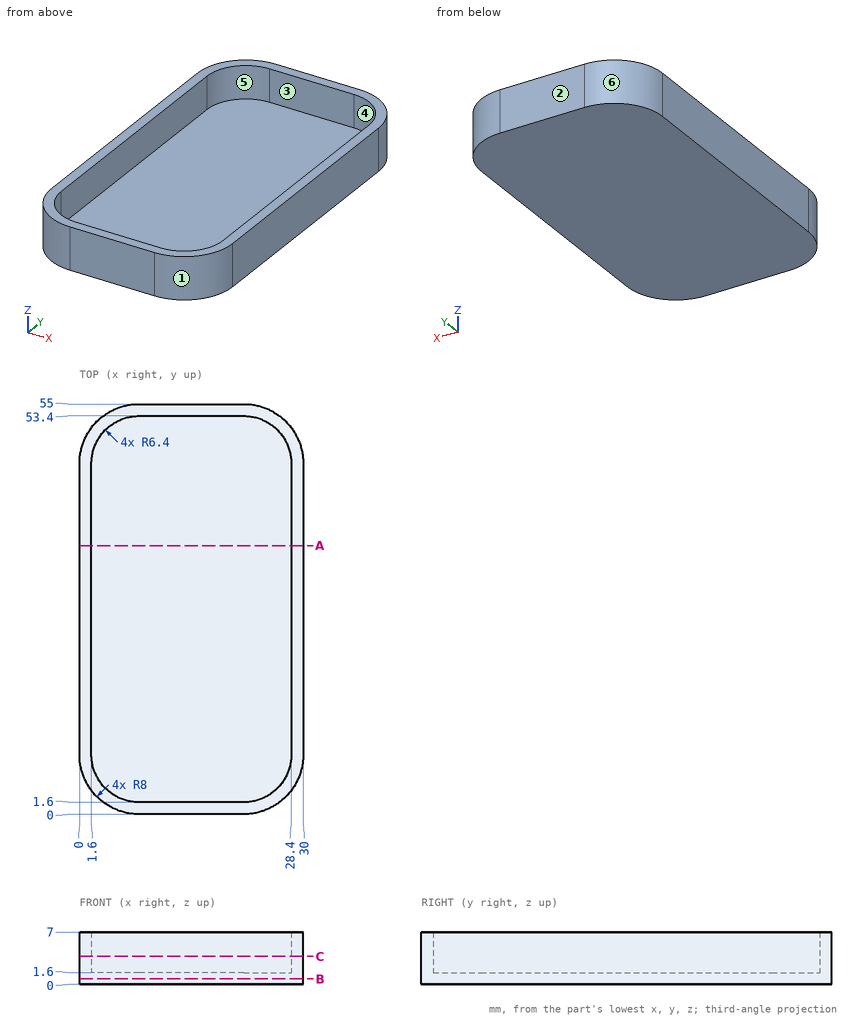
For this review, use the dimensioned drawing (mm, ordinates from the lowest corner) and the shaded views. A direction names the side the tool comes from. Round coordinates to 2 decimals unless told otherwise and drop trailing zeros. Write each loop counter-clockwise with the first axis right and the second up, starting at its lowest first coordinate (ties: lowest second). Pieces come first, ordered by that corner, then holes. Notation, with made-up numbers: (13.25, 46.25) -> (59.25, 46.25) arc R10 ccw to (59.25, 53.25) -> close; hole circle Ø11 at (-24, 75). An arc over 180 degrees is marked (long way). Use CSV: the item, a comma, the result in double quotes.
(1) Draft analysis for pull direction Y (two halves, no side actions). For the marked faces 1, 2, 3 and 4, state which applies: +Y half, -Y half, draft (parallel to the pull), parting line (faces both ways), or undercut.
Computed values:
face 1,"-Y half"
face 2,"+Y half"
face 3,"undercut"
face 4,"undercut"
(2) For the marked faces 5 and 6, list the 3-axis set-ups (+Z, -Z, +X, -X, +Y, -Y) from which the entire face can be reached by the end or side of a thin tool; tool diameter is ignored.
Computed values:
face 5,"+Z"
face 6,"+Z, -Z, -X, +Y"
(3) Consider section A-A, the plane y = 36. Give the boundary of the cut face in (x, z).
Computed values:
outline,"(0, 0) -> (30, 0) -> (30, 7) -> (28.4, 7) -> (28.4, 1.6) -> (1.6, 1.6) -> (1.6, 7) -> (0, 7) -> close"
(4) To check wall thickness, follow L1, parallel to Y at x = 9.25, z = 2; L2, parallel to X at y = 10.5, z = 2.75; L3, parallel to Z at x = 23.25, y = 41.5. State the ranges of each line that lie inside material, in increasing order. Write a range as [from, to].
Computed values:
L1,"[0, 1.6], [53.4, 55]"
L2,"[0, 1.6], [28.4, 30]"
L3,"[0, 1.6]"
(5) Consider section C-C, the plane z = 3.75. Give the boundary of the cut face in (x, y).
Computed values:
outline,"(0, 8) arc R8 ccw to (8, 0) -> (22, 0) arc R8 ccw to (30, 8) -> (30, 47) arc R8 ccw to (22, 55) -> (8, 55) arc R8 ccw to (0, 47) -> close; hole (1.6, 8) arc R6.4 ccw to (8, 1.6) -> (22, 1.6) arc R6.4 ccw to (28.4, 8) -> (28.4, 47) arc R6.4 ccw to (22, 53.4) -> (8, 53.4) arc R6.4 ccw to (1.6, 47) -> close"
(6) Consider section B-B, the plane z = 0.75. Give the boundary of the cut face in (x, y), plus the area to 3 significant figures.
Computed values:
outline,"(0, 8) arc R8 ccw to (8, 0) -> (22, 0) arc R8 ccw to (30, 8) -> (30, 47) arc R8 ccw to (22, 55) -> (8, 55) arc R8 ccw to (0, 47) -> close"
area,"1,600 mm²"
